Can you work these out from the model? Positions are in its coordinate system, mm. Face numbers are marked on the shaded views. Give positions to 0.01 mm unless a question says otherwise; leave off trailing zeros. Loops run counter-clockwise (first coordinate to the right, second up) from the corner with the lowest first, then second, coordinate; pieces in that order, holes last. Notation, with made-up numbers: M 28,26 L 49,26 A10 cw 49,44 Z; hole C 57,53 d4. An arc over 180 degrees is marked long. Use CSV: the item, a comma, the result in double quotes.
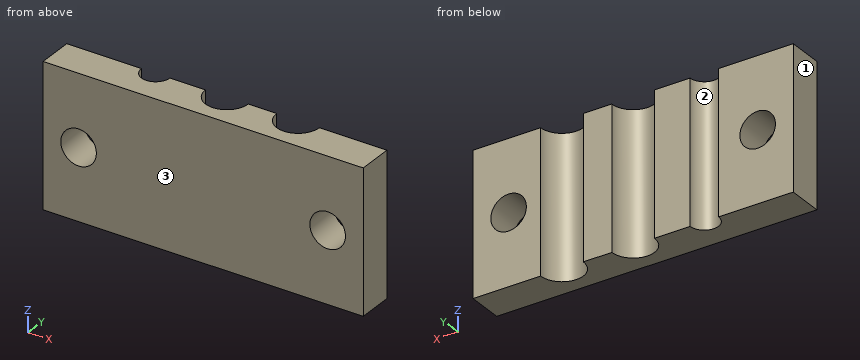
from build123d import *

# Parameters (mm, degrees)
BOSS_EXTRUDE1_DEPTH = 20
SKETCH2_R           = 2.5
CUT_EXTRUDE1_DEPTH  = 20
SKETCH3_W           = 45
SKETCH3_H           = 40
CUT_EXTRUDE2_DEPTH  = 20


with BuildPart() as part:
    # Sketch1 → Boss-Extrude1 (new body)
    with BuildSketch(Plane.XY):
        with BuildLine():
            Line((-22.5, -22.5), (22.5, -22.5))
            Line((22.5, -22.5), (22.5, 22.5))
            Line((22.5, 22.5), (13, 22.5))
            ThreePointArc((13, 22.5), (10, 19.5), (7, 22.5))
            Line((7, 22.5), (3, 22.5))
            ThreePointArc((3, 22.5), (0, 19.5), (-3, 22.5))
            Line((-3, 22.5), (-8, 22.5))
            ThreePointArc((-8, 22.5), (-10, 20.5), (-12, 22.5))
            Line((-12, 22.5), (-22.5, 22.5))
            Line((-22.5, 22.5), (-22.5, -22.5))
        make_face()
    extrude(amount=BOSS_EXTRUDE1_DEPTH)

    # Sketch2 → Cut-Extrude1 (cut)
    with BuildSketch(Plane(origin=(0, 22.5, 0), x_dir=(1, 0, 0), z_dir=(0, 1, 0))):
        with Locations((-17.5, -10)):
            Circle(SKETCH2_R)
        with Locations((17.5, -10)):
            Circle(SKETCH2_R)
    extrude(amount=-CUT_EXTRUDE1_DEPTH, mode=Mode.SUBTRACT)

    # Sketch3 → Cut-Extrude2 (cut)
    with BuildSketch(Plane(origin=(0, 0, 0), x_dir=(-1, 0, 0), z_dir=(0, 0, -1))):
        with Locations((0, -2.5)):
            Rectangle(SKETCH3_W, SKETCH3_H)
    extrude(amount=-CUT_EXTRUDE2_DEPTH, mode=Mode.SUBTRACT)


solid = part.part
Q1. I want a section at D-D, the plane y = 18.55. Please give me the cut outline in (x, z).
Model answer:
outline,"M -22.5,0 L 22.5,0 L 22.5,20 L -22.5,20 Z; hole C -17.5,10 d5; hole C 17.5,10 d5"
Q2. I want a section at C-C, the plane z = 1.75. Please give me the cut outline in (x, y).
Model answer:
outline,"M -22.5,17.5 L 22.5,17.5 L 22.5,22.5 L 13,22.5 A3 cw 7,22.5 L 3,22.5 A3 cw -3,22.5 L -8,22.5 A2 cw -12,22.5 L -22.5,22.5 Z"
Q3. Please list where these lines run through material, in increasing order: L1, parallel to X at y = 19, z = 10; L2, parallel to Z at x = 17.5, y = 19.7; L3, parallel to X at y = 19.95, z = 11.25. Write a range as from..to.
Model answer:
L1,"-22.5..-20, -15..15, 20..22.5"
L2,"0..7.5, 12.5..20"
L3,"-22.5..-19.67, -15.33..-1.58, 1.58..8.42, 11.58..15.33, 19.67..22.5"
Q4. If we mould it in two halves opening along X, with no side actions, what happens to the marked faces 1, 2 and 3? For each: released by +X, released by -X, zero draft, split by the parting line, or undercut.
Model answer:
face 1,"released by -X"
face 2,"undercut"
face 3,"zero draft"
Q5. I'm going to push a flat-ended pin straight in: P1, Ø3, axis at x = 17.5, z = 10, coming from the -Y side. Where does the tip first touch, or does it pass through?
Model answer:
P1,"through"
Q6. I want a section at B-B, the plane x = 17.5. Please give me the cut outline in (y, z), then the cut area to 3 significant figures.
Model answer:
outline,"M 17.5,0 L 22.5,0 L 22.5,7.5 L 17.5,7.5 Z; M 17.5,12.5 L 22.5,12.5 L 22.5,20 L 17.5,20 Z"
area,"75.0 mm2"
Q7. I want a section at A-A, the plane z = 8. Please give me the cut outline in (x, y).
Model answer:
outline,"M -22.5,17.5 L -19,17.5 L -19,22.5 L -22.5,22.5 Z; M -16,17.5 L 16,17.5 L 16,22.5 L 13,22.5 A3 cw 7,22.5 L 3,22.5 A3 cw -3,22.5 L -8,22.5 A2 cw -12,22.5 L -16,22.5 Z; M 19,17.5 L 22.5,17.5 L 22.5,22.5 L 19,22.5 Z"
